Autodesk Fusion 360 part; units mm, degrees
sketch "Sketch1" plane through (0, 0, 0) normal (0, 0, 1) x (1, 0, 0)
  circle A0 centre (0, 0) radius 2.45
  circle A1 centre (0, 0) radius 3.5
  circle A2 centre (0, 0) radius 4
  line L0 (0, 4) -> (-4, 4)
  arc A3 (-5, 5) -> (-4, 4) centre (-4, 5) ccw
  line L1 (-5, 5) -> (-5, 9)
  line L2 (-4, 11) -> (11.0351, 16.4723)
  line L3 (-4, 11) -> (12, 11) construction
  line L4 (0, -4) -> (-4, -4)
  line L5 (-10, 1.5) -> (-10, 10.4947)
  line L6 (-7, 15) -> (11.2229, 21.6326)
  arc A4 (-10, 1.5) -> (-4, -4) centre (-4, 2.0227) ccw
  arc A5 (-4, 11) -> (-5, 9) centre (-2.5, 9) ccw
  arc A6 (-7, 15) -> (-10, 10.4947) centre (-5.438, 10.7084) ccw
  line L7 (12.3, 16.7) -> (19.5014, 16.3173)
  line L8 (12.3, 21.7) -> (20, 21)
  line L9 (20, 16.7) -> (20.5, 20.5)
  arc A7 (20.5, 20.5) -> (20, 21) centre (19.95, 20.45) ccw
  arc A8 (19.5014, 16.3173) -> (20, 16.7) centre (19.527, 16.8001) ccw
  arc A9 (12.3, 21.7) -> (11.2229, 21.6326) centre (11.9798, 18.1776) ccw
  arc A10 (12.3, 16.7) -> (11.0351, 16.4723) centre (12.1512, 13.8992) ccw
  dimension "d1" = 4.9
  dimension "d2" = 7
  dimension "d3" = 8
  dimension "d4" = 4
  dimension "d6" = 20
  dimension "d7" = 16
sketch "Sketch2" plane through (0, 0, 4.5) normal (0, 0, 1) x (-1, 0, 0)
  line L0 (10, -10.4947) -> (10, -1.5)
  line L1 (4, 4) -> (0, 4)
  arc A0 (0, 4) -> (0, -4) centre (0, 0) ccw
  line L2 (0, -4) -> (4, -4)
  arc A1 (5, -5) -> (4, -4) centre (4, -5) ccw
  line L3 (5, -5) -> (5, -9)
  line L4 (4, -11) -> (-11.0351, -16.4723)
  line L5 (-11.2229, -21.6326) -> (7, -15)
  circle A2 centre (0, 0) radius 2.5
  circle A3 centre (0, 0) radius 1.1
  arc A4 (4, -11) -> (5, -9) centre (2.5, -9) ccw
  arc A5 (-12.3, -16.7) -> (-11.0351, -16.4723) centre (-12.1512, -13.8992) ccw
  line L6 (-12.3, -16.7) -> (-19.5014, -16.3173)
  arc A6 (-19.5014, -16.3173) -> (-20, -16.7) centre (-19.527, -16.8001) ccw
  line L7 (-20, -16.7) -> (-20.5, -20.5)
  arc A7 (-20.5, -20.5) -> (-20, -21) centre (-19.95, -20.45) ccw
  line L8 (-20, -21) -> (-12.3, -21.7)
  arc A8 (-12.3, -21.7) -> (-11.2229, -21.6326) centre (-11.9798, -18.1776) ccw
  arc A9 (7, -15) -> (10, -10.4947) centre (5.438, -10.7084) ccw
  arc A10 (10, -1.5) -> (4, 4) centre (4, -2.0227) ccw
  dimension "d14" = 5
  dimension "d15" = 2.2
extrude "Extrude5" add sketch "Sketch1" along normal blind 4.5 contours A0 | A1 | A2 | A2 L0 A3 L1 L2 L4 L5 L6 A4 A5 A6 L7 L8 L9 A7 A8 A9 A10
extrude "Extrude6" cut sketch "Sketch2" against normal blind 3.5 contours A2
extrude "Extrude7" cut sketch "Sketch2" against normal blind 5 contours A3
extrude "Extrude8" add sketch "Sketch1" against normal blind 3 contours A1
Geometry: final body of the model. Coordinates: model frame, mm. A direction names the side the tool comes from. Round coordinates to 2 decimals unless told otherwise and drop trailing zeros. Loops run counter-clockwise (first coordinate to the right, second up) from the corner with the lowest first, then second, coordinate; pieces in that order, holes last. Notation, with made-up numbers: (45, -33) - (50, -33) arc R3 ccw to (50, -29) - close; hole circle Ø10 at (33, 11.5). An arc over 180 degrees is marked (long way). Write each question's results on one line, items separated by ' | '. Start each with the question number.
1) Cut plane C-C on x = 2. Return loops of the section in (y, z).
2) Line query: probe 1 along Y at (x, z) = (0, 2.9); probe 2 along Y at (x, z) = (0, 0.7); probe 3 along Z at (x, y) = (3, 16). Output: solid intervals per line, ascending. Write a range as [from, to].
3) Cut plane D-D on z = 0.5. Return loops of the section in (x, y), then the cut area to 3 significant figures.
4) First-contact query: P1, Ø3, axis at x = 0, y = 0, coming from the +Z side; P2, Ø1.5, axis at y = 2, z = 1, coming from the -X side; P3, Ø3, axis at x = 0, y = 0, coming from the -Z side. Flat tips, straight axial feed; report the tip coordinate or a pass-through.
5) Cut plane B-B on y = 0. Return loops of the section in (x, z), then the cut area to 3 significant figures.
6) Access query for faces 4 (the face through (-5, 7, 2)), 5 (the face through (0.54, 2.44, 2.77)), 6 (the face through (15.85, 16.51, 2.22)), 7 (the face through (-0.5, -2.4, -1.5)), 8 (the face through (-8.02, -2.46, 2.22)). Directions: +Z, -Z, +X, -X, +Y, -Y. A direction counts if a zero-diameter tool reaches every point of the face in a straight line with its end or side. Return the directions, or none.
7) Mould query, pull axis X, two halves, no side actions, for faces 1 (the face through (-2, 12, 4.5)), 2 (the face through (-1, 1, 1)), 3 (the face through (11.751, 21.707, 2.218)). Classes: released by +X, released by -X, zero draft, split by the parting line, or undercut.
8) Cut plane A-A on z = 2. Return loops of the section in (x, y), then the cut area to 3 significant figures.
Verdict:
1) outline: (-3.46, 0) - (-2.87, 0) - (-2.87, -3) - (-1.42, -3) - (-1.42, 0) - (1.42, 0) - (1.42, -3) - (2.87, -3) - (2.87, 0) - (3.46, 0) - (3.46, 4.5) - (1.5, 4.5) - (1.5, 1) - (-1.5, 1) - (-1.5, 4.5) - (-3.46, 4.5) - close; (13.18, 0) - (18.28, 0) - (18.28, 4.5) - (13.18, 4.5) - close
2) probe 1: y = [-4, -2.5], [2.5, 4], [12.46, 17.55] | probe 2: y = [-4, -1.1], [1.1, 4], [12.46, 17.55] | probe 3: z = [0, 4.5]
3) outline: (-10, 1.5) arc R6.02 ccw to (-4, -4) - (0, -4) arc R4 ccw to (0, 4) - (-4, 4) arc R1 cw to (-5, 5) - (-5, 9) arc R2.5 cw to (-4, 11) - (11.04, 16.47) arc R2.8 cw to (12.3, 16.7) - (19.5, 16.32) arc R0.48 ccw to (20, 16.7) - (20.5, 20.5) arc R0.55 ccw to (20, 21) - (12.3, 21.7) arc R3.54 ccw to (11.22, 21.63) - (-7, 15) arc R4.57 ccw to (-10, 10.49) - close; hole circle Ø2.2 at (0, 0) | area: 273 mm2
4) P1: stops at z = 1 | P2: stops at x = -10 | P3: stops at z = 0
5) outline: (-9.67, 0) - (-3.5, 0) - (-3.5, -3) - (-2.45, -3) - (-2.45, 0) - (-1.1, 0) - (-1.1, 1) - (-2.5, 1) - (-2.5, 4.5) - (-9.67, 4.5) - close; (1.1, 0) - (2.45, 0) - (2.45, -3) - (3.5, -3) - (3.5, 0) - (4, 0) - (4, 4.5) - (2.5, 4.5) - (2.5, 1) - (1.1, 1) - close | area: 48.1 mm2
6) face 4: +Z, -Z, +X | face 5: +Z | face 6: +Z, -Z, -Y | face 7: -Z | face 8: +Z, -Z, -X, -Y
7) face 1: zero draft | face 2: undercut | face 3: split by the parting line
8) outline: (-10, 1.5) arc R6.02 ccw to (-4, -4) - (0, -4) arc R4 ccw to (0, 4) - (-4, 4) arc R1 cw to (-5, 5) - (-5, 9) arc R2.5 cw to (-4, 11) - (11.04, 16.47) arc R2.8 cw to (12.3, 16.7) - (19.5, 16.32) arc R0.48 ccw to (20, 16.7) - (20.5, 20.5) arc R0.55 ccw to (20, 21) - (12.3, 21.7) arc R3.54 ccw to (11.22, 21.63) - (-7, 15) arc R4.57 ccw to (-10, 10.49) - close; hole circle Ø5 at (0, 0) | area: 257 mm2
